CAD build for the part. Positions are in the model's coordinates, mm. Give positions to 0.01 mm unless a question says otherwise; leave off trailing zeros. Order: outer loops, then holes, each group sorted by start corner. A loop starts at its lowest first (then second) coordinate and runs counter-clockwise, first axis right, second up. Notation, with made-up numbers: (57, 48) -> (74, 48) arc R25 ccw to (74, 64) -> close; hole circle Ø11 at (37.25, 86). An arc over 180 degrees is marked (long way). Use one line per item in the form item = value. Start each with the question number.
1) Cut at C-C, the plane y = 2.35. State how many separate pieces and enclosed holes the cut face has, and give its area (3 significant figures).
2) Cut at A-A, the plane x = -22. Give the cut face in (y, z), and give its area (3 significant figures).
3) Drop flat-ended pins along their axis: P1, Ø0.9, axis at x = -35.5, y = 1.5, coming from the -Z side; P2, Ø1.5, axis at y = 1.5, z = 67, coming from the -X side; P3, Ø1.5, axis at y = 1.5, z = -46.5, coming from the +X side. Give the stop position or say it passes through.
4) Cut at B-B, the plane z = 4.5. Give the cut face in (x, y).
5) Probe line 1 (Z direction, x = -34.5, y = 1.4); line 2 (X direction, y = 0.5, z = 12.5); line 3 (Z direction, x = 25.5, y = 1.4). List the from-to ranges inside material, lowest first.
from build123d import *

# Parameters (mm, degrees)
BOSS_EXTRUDE1_DEPTH = 3
SKETCH2_R           = 1.6
CUT_EXTRUDE1_DEPTH  = 121.203993278
CHAMFER1_SIZE       = 1.5


with BuildPart() as part:
    # Sketch1 → Boss-Extrude1 (new body)
    with BuildSketch(Plane(origin=(0, 0, 0), x_dir=(1, 0, 0), z_dir=(0, 1, 0))):
        Polygon((-38, -114), (-12.666666667, -114), (-12.666666667, -109), (0, -109), (0, 114), (-12.666666667, 114), (-12.666666667, 109), (-33, 109), (-33, 85.5), (-38, 85.5), (-38, 57), (-33, 57), (-33, 28.5), (-38, 28.5), (-38, 0), (-33, 0), (-33, -28.5), (-38, -28.5), (-38, -57), (-33, -57), (-33, -85.5), (-38, -85.5), align=None)
    boss_extrude1 = extrude(amount=BOSS_EXTRUDE1_DEPTH)

    # Mirror1: Boss-Extrude1 across plane
    add(boss_extrude1.mirror(Plane(origin=(0, 3, 109), x_dir=(0, 0, 1), z_dir=(-1, 0, 0))))

    # Sketch2 → Cut-Extrude1 (cut, through all)
    with BuildSketch(Plane(origin=(0, 3, 0), x_dir=(1, 0, 0), z_dir=(0, 1, 0))):
        with Locations(Location((0, -85.5, 0), (0, 0, 270))):
            Circle(SKETCH2_R)
        with Locations(Location((0, -12.5, 0), (0, 0, 270))):
            Circle(SKETCH2_R)
    extrude(amount=-CUT_EXTRUDE1_DEPTH, mode=Mode.SUBTRACT)

    # Chamfer1
    chamfer1_edges = [part.edges().sort_by_distance(p)[0] for p in [
        (0, 3, 83.9),
        (0, 3, 10.9),
    ]]
    chamfer(chamfer1_edges, length=CHAMFER1_SIZE)


solid = part.part
Result:
q1.separate_pieces = 1
q1.enclosed_holes = 2
q1.area = 15,800 mm²
q2.outline = (0, -109) -> (3, -109) -> (3, 114) -> (0, 114) -> close
q2.area = 669 mm²
q3.P1 = -85.5
q3.P2 = -33
q3.P3 = 33
q4.outline = (-33, 0) -> (33, 0) -> (33, 3) -> (-33, 3) -> close
q5.line_1 = -85.5 to -57, -28.5 to 0, 28.5 to 57, 85.5 to 114
q5.line_2 = -33 to -1.6, 1.6 to 33
q5.line_3 = -109 to 114
